For this review, take the finished solid that the model builds, in its own axes (mm). Face numbers are marked on the shaded views. A direction names the side the tool comes from. Coordinates: 2 decimals unless noted, no trailing zeros. Write each loop counter-clockwise with the first axis right and the second up, starting at its lowest first coordinate (ties: lowest second). Pieces come first, ordered by that corner, then holes. Notation, with made-up numbers: M 20.25,71.25 L 43.25,71.25 A15 ccw 43.25,92.25 Z; hole C 50,-35 d7. An arc over 180 degrees is marked long. Return JSON: item names as keys, results as strings.
```python
from build123d import *

# Parameters (mm, degrees)
F0_R     = 5
F1_DEPTH = 15
F3_DEPTH = 5
F4_DEPTH = 25
F6_DEPTH = 10


with BuildPart() as f1:
    # F0 (on Top) → F1 (new body)
    with BuildSketch(Plane.XY):
        with BuildLine():
            ThreePointArc((0, -10), (7.0710678119, -7.0710678119), (10, 0))
            ThreePointArc((10, 0), (7.0710678119, 7.0710678119), (0, 10))
            ThreePointArc((0, 10), (-10, 0), (0, -10))
        make_face()
        Circle(F0_R, mode=Mode.SUBTRACT)
        with BuildLine():
            ThreePointArc((0, 10), (7.0710678119, 7.0710678119), (10, 0))
            ThreePointArc((10, 0), (7.0710678119, -7.0710678119), (0, -10))
            Line((0, -10), (15, -10))
            Line((15, -10), (20, -5))
            Line((20, -5), (20, 5))
            Line((20, 5), (15, 10))
            Line((15, 10), (0, 10))
        make_face()
    extrude(amount=F1_DEPTH)

    # F2 (on face) → F3 (join)
    with BuildSketch(Plane(origin=(0, 0, 0), x_dir=(1, 0, 0), z_dir=(0, 0, -1))):
        with BuildLine():
            ThreePointArc((0, 10), (-10, 0), (0, -10))
            Line((0, -10), (10, -10))
            Line((10, -10), (10, 10))
            Line((10, 10), (0, 10))
        make_face()
    extrude(amount=F3_DEPTH)

    # F4 (cut): a face of the model
    f4_faces = [f1.faces().sort_by_distance(p)[0] for p in [
        (0, 0, 0),
    ]]
    extrude(f4_faces, amount=-F4_DEPTH, mode=Mode.SUBTRACT)

    # F5 (on face) → F6 (cut)
    with BuildSketch(Plane.XY.offset(15)):
        with BuildLine():
            ThreePointArc((-9.6824583655, 2.5), (-10, 0), (-9.6824583655, -2.5))
            Line((-9.6824583655, -2.5), (20, -2.5))
            Line((20, -2.5), (20, 2.5))
            Line((20, 2.5), (-9.6824583655, 2.5))
        make_face()
    extrude(amount=-F6_DEPTH, mode=Mode.SUBTRACT)


solid = f1.part
```
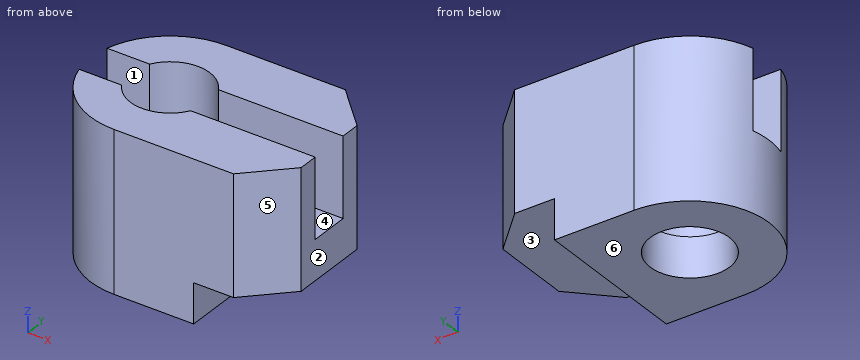
1. We need section B-B (y = 0). State the section outline as (x, z) points.
Checks:
{"outline": "M -10,-5 L -5,-5 L -5,5 L -10,5 Z; M 5,-5 L 10,-5 L 10,0 L 20,0 L 20,5 L 5,5 Z"}
2. We need section C-C (x = 11.5). State the section outline as (y, z) points, plus the area to 3 significant figures.
Checks:
{"outline": "M -10,0 L 10,0 L 10,15 L 2.5,15 L 2.5,5 L -2.5,5 L -2.5,15 L -10,15 Z", "area": "250 mm2"}
3. We need section A-A (z = 4). State the section outline as (x, y) points.
Checks:
{"outline": "M 0,-10 L 15,-10 L 20,-5 L 20,5 L 15,10 L 0,10 A10 ccw Z; hole C 0,0 d10"}
4. For the marked faces 1, 2 and 3, list the 3-axis set-ups (+Z, -Z, +X, -X, +Y, -Y) from which the entire face can be reached by the end or side of a thin tool; tool diameter is ignored.
Checks:
{"face 1": "+Z, +X, -X", "face 2": "+Z, -Z, +X, +Y, -Y", "face 3": "-Z, +X, +Y, -Y"}
5. Wall thickness on L1, parallel to Y at x = 0, z = 11; L2, parallel to Y at x = 6, z = 12; L3, parallel to Z at x = 14.75, y = 6.5: over which ranges is each line inside the solid? List them lowest first. Write a range as from..to.
Checks:
{"L1": "-10..-5, 5..10", "L2": "-10..-2.5, 2.5..10", "L3": "0..15"}
6. Draft analysis for pull direction Y (two halves, no side actions). For the marked faces 4, 5 and 6, state which applies: +Y half, -Y half, draft (parallel to the pull), parting line (faces both ways), or undercut.
Checks:
{"face 4": "undercut", "face 5": "-Y half", "face 6": "draft"}
7. We need section D-D (x = -2.5). State the section outline as (y, z) points.
Checks:
{"outline": "M -9.68,-5 L -4.33,-5 L -4.33,15 L -9.68,15 Z; M 4.33,-5 L 9.68,-5 L 9.68,15 L 4.33,15 Z"}
8. Clearance check with flat-ended pins moving along their axes: pin 1 Ø1.5 at (x, y) = (-7, 0.5) entering from +Z; pin 2 Ø1.6 at (x, z) = (-6.5, 9) entering from -Y; pin 3 Ø9 at (x, y) = (0, 0) entering from +Z; pin 4 Ø11 at (x, y) = (16, 4.5) entering from -Z. State where each tip first meets the part, or that it passes through.
Checks:
{"pin 1": "z = 5", "pin 2": "y = -8.22", "pin 3": "through", "pin 4": "z = 0"}
